Read the model definition and answer for the solid it produces. Units are mm, in the model's axes. Face numbers are marked on the shaded views. A direction names the side the tool comes from. Round coordinates to 2 decimals unless told otherwise and drop trailing zeros. Write each loop counter-clockwise with the first axis right and the second up, starting at its lowest first coordinate (ties: lowest second). Pieces come first, ordered by that corner, then holes. Notation, with made-up numbers: (19.25, 73.5) - (57.25, 73.5) arc R34 ccw to (57.25, 110.5) - close; hole circle Ø1 at (-26, 37.25). An arc over 180 degrees is marked (long way). One line per item, written item: value. Start each with the question number.
(1) The mould has two halves that part along X. Classify the marked faces 1, 2 and 3: +X half, -X half, draft (parallel to the pull), parting line (faces both ways), or undercut.
(2) Flat-ended cylindrical pins translate along their axes: pin 1 Ø9 at (x, z) = (89, -65) entering from +Y; pin 2 Ø8 at (x, z) = (12.7, -12.7) entering from +Y; pin 3 Ø5 at (y, z) = (36.5, -28.5) entering from -X. Find the tip coordinate at first contact, or state that the pin passes through.
(3) For the marked faces 4, 5, 6 and 7, determine the directions among +Z, -Z, +X, -X, +Y, -Y from which every point of the face is accessible in a straight line to the end or side of a thin tool.
(4) A cutting plane is placed at A-A, the plane z = -62. Determine the outline of the cut face in (x, y), plus the area to 3 significant figures.
(5) Find the intervals of material crossed by L1, parallel to X at y = 10, z = -12.7; L2, parallel to Y at x = 68, z = -59.5; L3, parallel to Y at x = 84.5, z = -60.5, in increasing order.
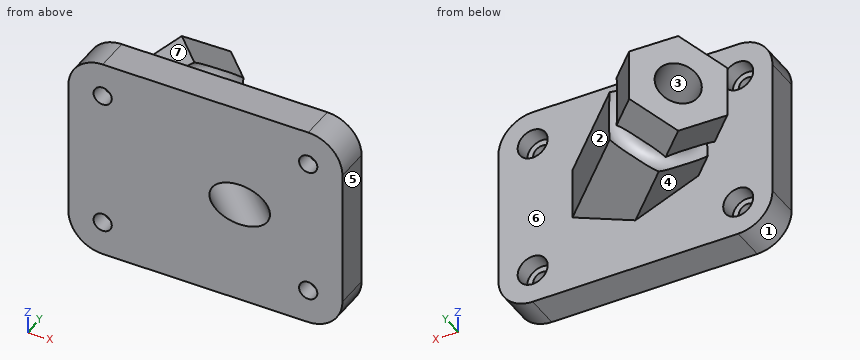
from build123d import *

# Parameters (mm, degrees)
BOSS_EXTRUDE1_DEPTH                                 = 12.7
CBORE_FOR_00_BINDING_HEAD_MACHINE_SCREW_D           = 6.7564
CBORE_FOR_00_BINDING_HEAD_MACHINE_SCREW_CBORE_D     = 11.1252
CBORE_FOR_00_BINDING_HEAD_MACHINE_SCREW_CBORE_DEPTH = 6.35
BOSS_EXTRUDE2_DEPTH                                 = 50.8
BOSS_EXTRUDE2_DEPTH_BACK                            = 50.8
SKETCH10_R                                          = 4.7752
SKETCH11_R                                          = 7.9375
CUT_EXTRUDE1_DEPTH                                  = 148.399953238


with BuildPart() as part:
    # Sketch1 → Boss-Extrude1 (new body)
    with BuildSketch(Plane(origin=(0, 0, 0), x_dir=(1, 0, 0), z_dir=(0, 1, 0))):
        with BuildLine():
            Line((12.7, 0), (88.9, 0))
            ThreePointArc((88.9, 0), (97.880256121, 3.719743879), (101.6, 12.7))
            Line((101.6, 12.7), (101.6, 63.5))
            ThreePointArc((101.6, 63.5), (97.880256121, 72.480256121), (88.9, 76.2))
            Line((88.9, 76.2), (12.7, 76.2))
            ThreePointArc((12.7, 76.2), (3.719743879, 72.480256121), (0, 63.5))
            Line((0, 63.5), (0, 12.7))
            ThreePointArc((0, 12.7), (3.719743879, 3.719743879), (12.7, 0))
        make_face()
    extrude(amount=BOSS_EXTRUDE1_DEPTH)

    # CBORE for #00 Binding Head Machine Screw1 (through all)
    with Locations(Plane(origin=(12.7, 12.7, -12.7), x_dir=(0, 0, 1), z_dir=(0, 1, 0))):
        with Locations((0, 0), (0, 76.2), (-50.8, 76.2), (-50.8, 0)):
            CounterBoreHole(CBORE_FOR_00_BINDING_HEAD_MACHINE_SCREW_D / 2, CBORE_FOR_00_BINDING_HEAD_MACHINE_SCREW_CBORE_D / 2, CBORE_FOR_00_BINDING_HEAD_MACHINE_SCREW_CBORE_DEPTH)


with BuildPart() as body_2:
    # Sketch7 → Boss-Extrude2 (new, two sides: drawn at the far end of the back side and taken through both)
    with BuildSketch(Plane(origin=(19.05, -19.05, 0), x_dir=(0, 0, 1), z_dir=(-0.7071067811865488, 0.7071067811865464, 0)).offset(-BOSS_EXTRUDE2_DEPTH_BACK)):
        Polygon((-57.15, 44.901280605), (-47.625, 28.403496663), (-28.575, 28.403496663), (-19.05, 44.901280605), (-28.575, 61.399064547), (-47.625, 61.399064547), align=None)
    extrude(amount=BOSS_EXTRUDE2_DEPTH + BOSS_EXTRUDE2_DEPTH_BACK)

    # SurfaceCut16: cut with a surface, the side behind it stays
    # Surface-Offset1: a surface, a copy of 1 face of the part
    surface_offset1_1 = part.part.faces().sort_by_distance((50.8, 0, -38.1))[0]
    split(bisect_by=surface_offset1_1, keep=Keep.BOTTOM)

    # Sketch10 → Cut-Revolve1 (revolve, cut)
    with BuildSketch(Plane(origin=(0, 0, -38.1), x_dir=(-1, 0, 0), z_dir=(0, 0, -1)), mode=Mode.PRIVATE) as cut_revolve1_sk:
        with Locations((-40.015054597, 46.816335203)):
            Circle(SKETCH10_R)
    revolve(cut_revolve1_sk.sketch.rotate(Axis((14.878975516, 48.621024484, -38.1), (0.7071067811865499, -0.7071067811865451, 0)), 150.000000006), axis=Axis((14.878975516, 48.621024484, -38.1), (0.7071067811865499, -0.7071067811865451, 0)), mode=Mode.SUBTRACT)


with BuildPart() as cut_extrude1_tool:
    # Sketch11 → Cut-Extrude1 (new, through all)
    with BuildSketch(Plane(origin=(-16.871024484, 16.871024484, 0), x_dir=(0, 0, 1), z_dir=(-0.7071067811865488, 0.7071067811865462, 0))):
        with Locations(Location((-38.1, 44.901280605, 0), (0, 0, 270))):
            Circle(SKETCH11_R)
    extrude(amount=-CUT_EXTRUDE1_DEPTH)


with BuildPart() as part_1:
    add(part.part)

    # Cut-Extrude1: cut by cut_extrude1_tool
    add(cut_extrude1_tool.part, mode=Mode.SUBTRACT)


with BuildPart() as body_2_1:
    add(body_2.part)

    # Cut-Extrude1: cut by cut_extrude1_tool
    add(cut_extrude1_tool.part, mode=Mode.SUBTRACT)


with BuildPart() as part_2:
    add(part_1.part)

    # Combine1: union body 2
    add(body_2_1.part)


solid = part_2.part
Here are the results:
1. face 1: -X half
1. face 2: +X half
1. face 3: undercut
2. pin 1: y = 12.7
2. pin 2: y = 6.35
2. pin 3: x = 3.21
3. face 4: -Z, -X
3. face 5: +Z, -Z, +X, +Y, -Y
3. face 6: none
3. face 7: +Z, -X
4. outline: (0, 0) - (9.67, 0) - (9.67, 6.35) - (7.34, 6.35) - (7.34, 12.7) - (0, 12.7) - close; (15.73, 0) - (85.87, 0) - (85.87, 6.35) - (83.54, 6.35) - (83.54, 12.7) - (18.06, 12.7) - (18.06, 6.35) - (15.73, 6.35) - close; (91.93, 0) - (101.6, 0) - (101.6, 12.7) - (94.26, 12.7) - (94.26, 6.35) - (91.93, 6.35) - close
4. area: 1,080 mm²
5. L1: 0 to 7.14, 18.26 to 83.34, 94.46 to 101.6
5. L2: 0 to 12.7
5. L3: 0 to 6.35
